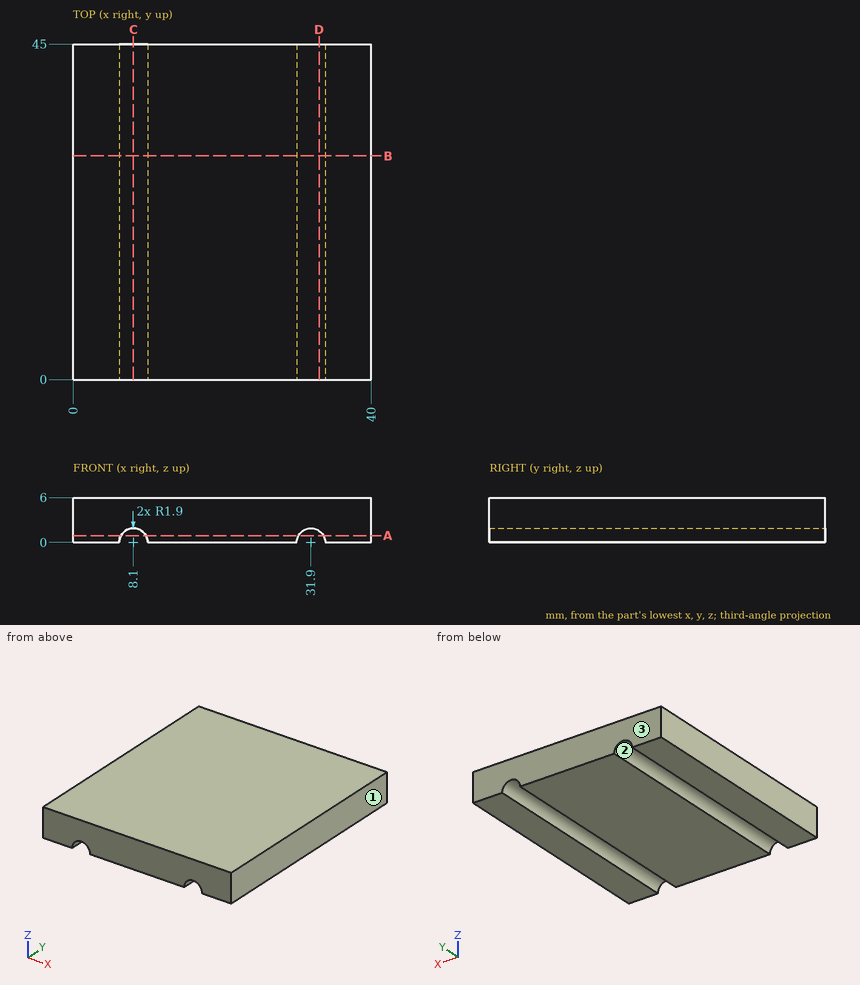
Verification items for this drawing (mm, ordinates from the low corner). Coordinates: 2 decimals unless noted, no trailing zeros. Write each loop counter-clockwise with the first axis right and the second up, starting at its lowest first coordinate (ties: lowest second). Pieces come first, ordered by that corner, then holes. Notation, with made-up numbers: (-18, 62.25) - (39, 62.25) arc R23 ccw to (39, 81.25) - close; hole circle Ø10 at (10, 21). An arc over 180 degrees is marked (long way). One line per question, with ' | ' between items.
Item 1: Thickness scan on line 1 (Z direction, x = 8, y = 3); line 2 (Z direction, x = 7, y = 15.5). Record the ranges inside material, lowest first. Write a range as [from, to].
Determined:
line 1: z = [1.9, 6] | line 2: z = [1.55, 6]
Item 2: Sectioned sample at D-D on x = 33. Record the boundary of the cut face in (y, z).
Determined:
outline: (0, 1.55) - (45, 1.55) - (45, 6) - (0, 6) - close
Item 3: Mould release check, pull along X, two halves, no side actions. Record for the marked faces 1, 2 and 3: pulls with the +X half, pulls with the -X half, needs draft (parallel to the pull), parting line crosses it, or undercut.
Determined:
face 1: pulls with the +X half | face 2: undercut | face 3: needs draft
Item 4: Sectioned sample at C-C on x = 8.1. Record the boundary of the cut face in (y, z), plus the area to 4 significant figures.
Determined:
outline: (0, 1.9) - (45, 1.9) - (45, 6) - (0, 6) - close | area: 184.5 mm2
Item 5: Sectioned sample at A-A on z = 0.9. Record the boundary of the cut face in (x, y).
Determined:
outline: (0, 0) - (6.43, 0) - (6.43, 45) - (0, 45) - close; (9.77, 0) - (30.23, 0) - (30.23, 45) - (9.77, 45) - close; (33.57, 0) - (40, 0) - (40, 45) - (33.57, 45) - close
Item 6: Sectioned sample at B-B on y = 30. Record the boundary of the cut face in (x, z).
Determined:
outline: (0, 0) - (6.2, 0) arc R1.9 cw to (10, 0) - (30, 0) arc R1.9 cw to (33.8, 0) - (40, 0) - (40, 6) - (0, 6) - close
